```python
from build123d import *

# Parameters (mm, degrees)
SKETCH1_W             = 8.255
SKETCH1_H             = 22.225
BOSS_EXTRUDE1_DEPTH   = 6.35
SKETCH2_W             = 6.35
SKETCH2_H             = 4.7625
BOSS_EXTRUDE2_DEPTH   = 6.35
BOSS_EXTRUDE3_START   = -8.255
SKETCH2_4_W           = 6.35
SKETCH2_4_H           = 4.7625
BOSS_EXTRUDE3_DEPTH   = 6.35
F_4_CLEARANCE_HOLE1_D = 3.4544
F_4_CLEARANCE_HOLE2_D = 3.4544
CHAMFER1_SIZE         = 3.175
CHAMFER2_SIZE         = 0.762


with BuildPart() as part:
    # Sketch1 → Boss-Extrude1 (new body)
    with BuildSketch(Plane.XY):
        with Locations((-55.673222486, -11.1125)):
            Rectangle(SKETCH1_W, SKETCH1_H)
    extrude(amount=BOSS_EXTRUDE1_DEPTH)

    # Sketch2 → Boss-Extrude2 (add)
    with BuildSketch(Plane.ZY.offset(59.800722486)):
        with Locations((3.175, -2.38125)):
            Rectangle(SKETCH2_W, SKETCH2_H)
    extrude(amount=BOSS_EXTRUDE2_DEPTH)

    # Sketch2<4> → Boss-Extrude3 (add)
    with BuildSketch(Plane.ZY.offset(59.800722486).offset(BOSS_EXTRUDE3_START)):
        with Locations((3.175, -2.38125)):
            Rectangle(SKETCH2_4_W, SKETCH2_4_H)
    extrude(amount=-BOSS_EXTRUDE3_DEPTH)

    # #4 Clearance Hole1 (through all)
    with Locations(Plane(origin=(0, 0, 0), x_dir=(-1, 0, 0), z_dir=(0, 0, -1))):
        with Locations((55.673222486, -6.35)):
            Hole(F_4_CLEARANCE_HOLE1_D / 2)

    # Sketch6 → Hole1 (revolve, cut)
    with BuildSketch(Plane(origin=(-55.673222486, -6.35, 0), x_dir=(0, 1, 0), z_dir=(1, 0, 0))):
        Polygon((0, 0), (0, 3.429), (1.9431, 3.429), (2.0701, 0), align=None)
    revolve(axis=Axis((-55.673222486, -6.35, 110), (0, 0, -1)), mode=Mode.SUBTRACT)

    # #4 Clearance Hole2 (through all)
    with Locations(Plane(origin=(0, -4.7625, 0), x_dir=(-1, 0, 0), z_dir=(0, -1, 0))):
        with Locations((48.370722486, -3.175), (62.975722486, -3.175)):
            Hole(F_4_CLEARANCE_HOLE2_D / 2)

    # Chamfer1
    chamfer1_edges = [part.edges().sort_by_distance(p)[0] for p in [
        (-55.673222486, -22.225, 6.35),
    ]]
    chamfer(chamfer1_edges, length=CHAMFER1_SIZE)

    # Chamfer2
    chamfer2_edges = [part.edges().sort_by_distance(p)[0] for p in [
        (-59.800722486, -13.49375, 0),
        (-59.800722486, -11.90625, 6.35),
        (-62.975722486, -4.7625, 6.35),
        (-62.975722486, -4.7625, 0),
        (-66.150722486, -2.38125, 6.35),
        (-55.673222486, 0, 6.35),
        (-66.150722486, 0, 3.175),
        (-66.150722486, -2.38125, 0),
        (-66.150722486, -4.7625, 3.175),
        (-45.195722486, -2.38125, 0),
        (-48.370722486, -4.7625, 0),
        (-45.195722486, 0, 3.175),
        (-48.370722486, -4.7625, 6.35),
        (-45.195722486, -2.38125, 6.35),
        (-45.195722486, -4.7625, 3.175),
        (-55.673222486, 0, 0),
        (-51.545722486, -13.49375, 0),
        (-51.545722486, -11.90625, 6.35),
        (-51.545722486, -22.225, 1.5875),
        (-51.545722486, -20.6375, 4.7625),
        (-59.800722486, -22.225, 1.5875),
        (-59.800722486, -20.6375, 4.7625),
    ]]
    chamfer(chamfer2_edges, length=CHAMFER2_SIZE)


solid = part.part
```
Here's how the part is built. I have some questions about the finished solid (model axes, mm). A direction names the side the tool comes from. Round coordinates to 2 decimals unless told otherwise and drop trailing zeros. Write each loop counter-clockwise with the first axis right and the second up, starting at its lowest first coordinate (ties: lowest second). Pieces come first, ordered by that corner, then holes.
Q1. If we section it at C-C on x = -47.5: Write out the boundary of the cut face in (y, z), plus the area to 3 significant figures.
Q2. If we section it at A-A on y = -6.35: Write out the boundary of the cut face in (x, z), plus the area to 3 significant figures.
Q3. If we section it at B-B on z = 4.5: Write out the boundary of the cut face in (x, y).
Q4. Please list where these lines run through material, in increasing order: probe 1 along Y at (x, z) = (-51.25, 1.5); probe 2 along X at (y, z) = (-17.75, 2); probe 3 along Z at (x, y) = (-63.75, -3.75).
Q5. If we section it at D-D on y = -8.75: Write out the boundary of the cut face in (x, z).
Q6. Which directions (+Z, -Z, +X, -X, +Y, -Y) give clear straight access to the entire face, cutting with the end or side of a thin tool? Please do faces 1 (the flat face through (-50, -4.762, 4.2)), 2 (the flat face through (-45.196, -2, 3)), 3 (the flat face through (-61, -4.762, 4)).
Q7. If we mould it in two halves opening along X, with no side actions, what happens to faces 4 (the cylindrical face through (-46.72, -2.35, 2.66)), 5 (the flat face through (-59.801, -13, 3)), 6 (the flat face through (-56, 0, 3))? For each: +X half, -X half, draft (parallel to the pull), parting line (faces both ways), or undercut.
Q8. Will these pins go through, and if not, where does the flat tip stop? P1, Ø3, axis at y = -13, z = 2, coming from the -X side; P2, Ø3, axis at x = -54.5, y = -6.5, coming from the -Z side; P3, Ø1.4, axis at y = -12.5, z = 2.5, coming from the +X side; P4, Ø2.5, axis at x = -64, z = 4, coming from the -Y side.
Answer below:
1. outline: (-4.76, 0.76) - (-4, 0) - (-0.76, 0) - (0, 0.76) - (0, 1.68) - (-4.76, 1.68) - close; (-4.76, 4.67) - (0, 4.67) - (0, 5.59) - (-0.76, 6.35) - (-4, 6.35) - (-4.76, 5.59) - close
1. area: 14.9 mm2
2. outline: (-59.8, 0.76) - (-59.04, 0) - (-57.74, 0) - (-57.62, 3.43) - (-57.4, 3.43) - (-57.4, 6.35) - (-59.04, 6.35) - (-59.8, 5.59) - close; (-53.95, 3.43) - (-53.73, 3.43) - (-53.6, 0) - (-52.31, 0) - (-51.55, 0.76) - (-51.55, 5.59) - (-52.31, 6.35) - (-53.95, 6.35) - close
2. area: 27.4 mm2
3. outline: (-66.15, -4) - (-65.39, -4.76) - (-64.08, -4.76) - (-64.08, 0) - (-65.39, 0) - (-66.15, -0.76) - close; (-61.87, -4.76) - (-59.8, -4.76) - (-59.8, -19.82) - (-59.04, -20.9) - (-52.31, -20.9) - (-51.55, -19.82) - (-51.55, -4.76) - (-49.48, -4.76) - (-49.48, 0) - (-61.87, 0) - close; (-47.26, -4.76) - (-45.96, -4.76) - (-45.2, -4) - (-45.2, -0.76) - (-45.96, 0) - (-47.26, 0) - close; hole circle Ø3.45 at (-55.67, -6.35)
4. probe 1: y = -4.76 to 0
4. probe 2: x = -59.8 to -51.55
4. probe 3: z = 0 to 1.63, 4.72 to 6.35
5. outline: (-59.8, 0.76) - (-59.04, 0) - (-52.31, 0) - (-51.55, 0.76) - (-51.55, 5.59) - (-52.31, 6.35) - (-59.04, 6.35) - (-59.8, 5.59) - close
6. face 1: +Z, -Z, +X, -Y
6. face 2: +Z, -Z, +X, +Y, -Y
6. face 3: +Z, -Z, -X, -Y
7. face 4: undercut
7. face 5: -X half
7. face 6: draft
8. P1: stops at x = -59.8
8. P2: stops at z = 0
8. P3: stops at x = -51.55
8. P4: stops at y = -4.76
